For this review, take the finished solid that the model builds, in its own axes (mm). Face numbers are marked on the shaded views. A direction names the side the tool comes from. Give positions to 0.01 mm unless a question says otherwise; leave off trailing zeros. Loops run counter-clockwise (first coordinate to the right, second up) from the corner with the lowest first, then second, coordinate; pieces in that order, holes last. Notation, with made-up numbers: (31, 21.25) - (62, 21.25) arc R19 ccw to (62, 25.25) - close; hole circle Ø2 at (-13.75, 19). An arc over 180 degrees is marked (long way). Put each result on its own line as item: value. Start each with the question number.
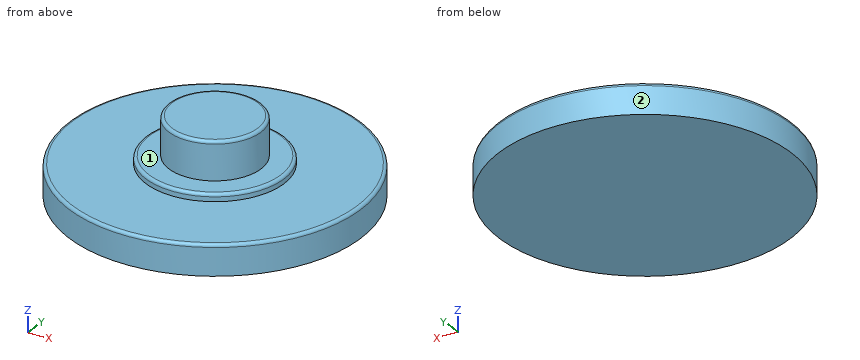
from build123d import *

# Parameters (mm, degrees)
F0_R     = 9.5
F1_DEPTH = 2
F2_R     = 4.5
F3_DEPTH = 0.5
F4_R     = 3
F5_DEPTH = 2.5
F6_R     = 0.2


with BuildPart() as f1:
    # F0 (on Top) → F1 (new body)
    with BuildSketch(Plane.XY):
        Circle(F0_R)
    extrude(amount=F1_DEPTH)

    # F2 (on face) → F3 (join)
    with BuildSketch(Plane.XY.offset(2)):
        Circle(F2_R)
    extrude(amount=F3_DEPTH)

    # F4 (on face) → F5 (join)
    with BuildSketch(Plane.XY.offset(2.5)):
        Circle(F4_R)
    extrude(amount=F5_DEPTH)

    # F6
    f6_edges = [f1.edges().sort_by_distance(p)[0] for p in [
        (-3, 0, 5),
        (-4.5, 0, 2.5),
        (-9.5, 0, 2),
    ]]
    fillet(f6_edges, radius=F6_R)


solid = f1.part
1) Machinability: for the marked faces 1 and 2, which of the approach directions +Z, -Z, +X, -X, +Y, -Y give a long, thin tool a straight path to every point of the face, cutting with its end or side? Answer none if there is none.
2) Wall thickness on probe 1 along Z at (x, y) = (-1, 5); probe 2 along Z at (x, y) = (3.25, 0); probe 3 along Y at (x, z) = (3.75, 1.8): over which ranges is each line inside the solid? List them lowest first.
3) Insertion check: P1, Ø1, axis at x = -7.5, z = 4, coming from the +Y side; P2, Ø2, axis at y = -3, z = 1.5, coming from the +X side; P3, Ø2, axis at x = 7, z = 0.5, coming from the -Y side; P4, Ø1.5, axis at y = -3, z = 2.5, coming from the +X side. Each pin has a flat end and moves straight along its axis. Give the tip position at first contact, or say it passes through.
4) Take a section at A-A on y = 0. State the section outline as (x, z) points, and give its area (3 significant figures).
5) Take a section at D-D on z = 3.9. State the section outline as (x, y) points, and give its area (3 significant figures).
6) Take a section at C-C on z = 0.75. State the section outline as (x, y) points.
Answers follow:
1. face 1: +Z
1. face 2: +Z, -Z
2. probe 1: 0 to 2
2. probe 2: 0 to 2.5
2. probe 3: -8.73 to 8.73
3. P1: through
3. P2: x = 9.29
3. P3: y = -7.37
3. P4: x = 9.13
4. outline: (-9.5, 0) - (9.5, 0) - (9.5, 1.8) arc R0.2 ccw to (9.3, 2) - (4.5, 2) - (4.5, 2.3) arc R0.2 ccw to (4.3, 2.5) - (3, 2.5) - (3, 4.8) arc R0.2 ccw to (2.8, 5) - (-2.8, 5) arc R0.2 ccw to (-3, 4.8) - (-3, 2.5) - (-4.3, 2.5) arc R0.2 ccw to (-4.5, 2.3) - (-4.5, 2) - (-9.3, 2) arc R0.2 ccw to (-9.5, 1.8) - close
4. area: 57.4 mm2
5. outline: circle Ø6 at (0, 0)
5. area: 28.3 mm2
6. outline: circle Ø19 at (0, 0)
